Source: CAD feature listing. Evaluate the final solid. Frame: model axes, mm. A direction names the side the tool comes from. Coordinates: 2 decimals unless noted, no trailing zeros. Order: outer loops, then holes, each group sorted by start corner. A loop starts at its lowest first (then second) coordinate and runs counter-clockwise, first axis right, second up. Notation, with made-up numbers: (78, 85) -> (133, 85) arc R15 cw to (133, 95) -> close; hole circle Ø10 at (64, 89.25). An arc over 180 degrees is marked (long way). Put each result on its own line as item: value.
from build123d import *

# Parameters (mm, degrees)
PAD_DEPTH       = 50
SKETCH001_R     = 3.35
POCKET_DEPTH    = 5.001
FILLET_R        = 10
SKETCH002_R     = 7
POCKET001_DEPTH = 3.001


with BuildPart() as part:
    # Sketch → Pad (new body)
    with BuildSketch(Plane.XY):
        with BuildLine():
            Line((0, 65), (0, 10))
            ThreePointArc((0, 10), (2.928932, 2.928932), (10, 0))
            Line((10, 0), (80, 0))
            Line((80, 0), (80, -5))
            Line((80, -5), (10, -5))
            ThreePointArc((-5, 10), (-0.606602, -0.606602), (10, -5))
            Line((-5, 10), (-5, 65))
            Line((-5, 65), (0, 65))
        make_face()
    extrude(amount=PAD_DEPTH)

    # Sketch001 → Pocket (cut, through all)
    with BuildSketch(Plane.YZ):
        with Locations((45, 25)):
            Circle(SKETCH001_R)
    extrude(amount=-POCKET_DEPTH, mode=Mode.SUBTRACT)

    # Fillet
    fillet_edges = [part.edges().sort_by_distance(p)[0] for p in [
        (-2.5, 65, 0),
        (-2.5, 65, 50),
        (80, -2.5, 50),
        (80, -2.5, 0),
    ]]
    fillet(fillet_edges, radius=FILLET_R)

    # Sketch002 → Pocket001 (cut, through all)
    with BuildSketch(Plane.YZ.offset(-2)):
        with Locations((45, 25)):
            Circle(SKETCH002_R)
    extrude(amount=-POCKET001_DEPTH, mode=Mode.SUBTRACT)


solid = part.part
1. Cut plane C-C on z = 15.5. Output: boundary loops of the cut face in (x, y), plus the area to 3 significant figures.
Numbers:
outline: (-5, 10) arc R15 ccw to (10, -5) -> (80, -5) -> (80, 0) -> (10, 0) arc R10 cw to (0, 10) -> (0, 65) -> (-5, 65) -> close
area: 723 mm2
2. Set-up query: faces 1 (the flat face through (0, 38, 25)), 2 (the cylindrical face through (-2.46, 62.15, 3.01)), 3 (the flat face through (-2, 43, 22)). Return all of +Z, -Z, +X, -X, +Y, -Y with unobstructed straight access to the full face (end or side cutting, diameter ignored); none if empty.
Numbers:
face 1: +Z, -Z, +X, +Y
face 2: -Z, +X, -X, +Y
face 3: -X
3. Cut plane D-D on x = 31. Output: boundary loops of the cut face in (y, z).
Numbers:
outline: (-5, 0) -> (0, 0) -> (0, 50) -> (-5, 50) -> close
4. Cut plane A-A on z = 25. Output: boundary loops of the cut face in (x, y).
Numbers:
outline: (-5, 10) arc R15 ccw to (10, -5) -> (80, -5) -> (80, 0) -> (10, 0) arc R10 cw to (0, 10) -> (0, 41.65) -> (-2, 41.65) -> (-2, 38) -> (-5, 38) -> close; (-5, 52) -> (-2, 52) -> (-2, 48.35) -> (0, 48.35) -> (0, 65) -> (-5, 65) -> close
5. Pull-direction query (Y, two-part tool) for faces 4 (the cylindrical face through (76.99, -2.54, 47.15)), 5 (the cylindrical face through (-3.48, 48.23, 18.79)), 6 (the cylindrical face through (-2.46, 62.15, 46.99)); classes: pulls with the +Y half, pulls with the -Y half, needs draft (parallel to the pull), parting line crosses it, or undercut.
Numbers:
face 4: needs draft
face 5: undercut
face 6: pulls with the +Y half
6. First-contact query: pin 1 (15 mm diameter, centred on y = 39.5, z = 18.5, fed in from +X); pin 2 (1 mm diameter, centred on x = 30.5, z = 18.5, fed in from +Y); pin 3 (1 mm diameter, centred on x = 7, z = 40.5, fed in from +Y); pin 4 (5.5 mm diameter, centred on y = 45, z = 25, fed in from +X). Flat tips, straight axial feed; report the tip coordinate or a pass-through.
Numbers:
pin 1: stops at x = 0
pin 2: stops at y = 0
pin 3: stops at y = 0.63
pin 4: passes through
7. Cut plane B-B on y = 45. Output: boundary loops of the cut face in (x, z).
Numbers:
outline: (-5, 0) -> (0, 0) -> (0, 21.65) -> (-2, 21.65) -> (-2, 18) -> (-5, 18) -> close; (-5, 32) -> (-2, 32) -> (-2, 28.35) -> (0, 28.35) -> (0, 50) -> (-5, 50) -> close
8. Ray query, line 1 along Z through (x, y) = (-3.5, 45); line 2 along Z through (x, y) = (-0.5, 45); line 3 along X through (y, z) = (23, 3.5). Return the intervals inside material, ascending.
Numbers:
line 1: z = 0 to 18, 32 to 50
line 2: z = 0 to 21.65, 28.35 to 50
line 3: x = -5 to 0
